Print and shaded views of the part. All mm, measured from the part's lowest x, y and z. A direction names the side the tool comes from. Round coordinates to 2 decimals unless told otherwise and drop trailing zeros. Order: outer loops, then holes, each group sorted by start corner. A loop starts at its lowest first (then second) coordinate and runs counter-clockwise, first axis right, second up. Notation, with made-up numbers: (-32.5, 1.25) - (-16.5, 1.25) arc R31 ccw to (-16.5, 35.25) - close; hole circle Ø3 at (3.5, 82.25). An arc over 180 degrees is marked (long way). Write item = value, one per line.
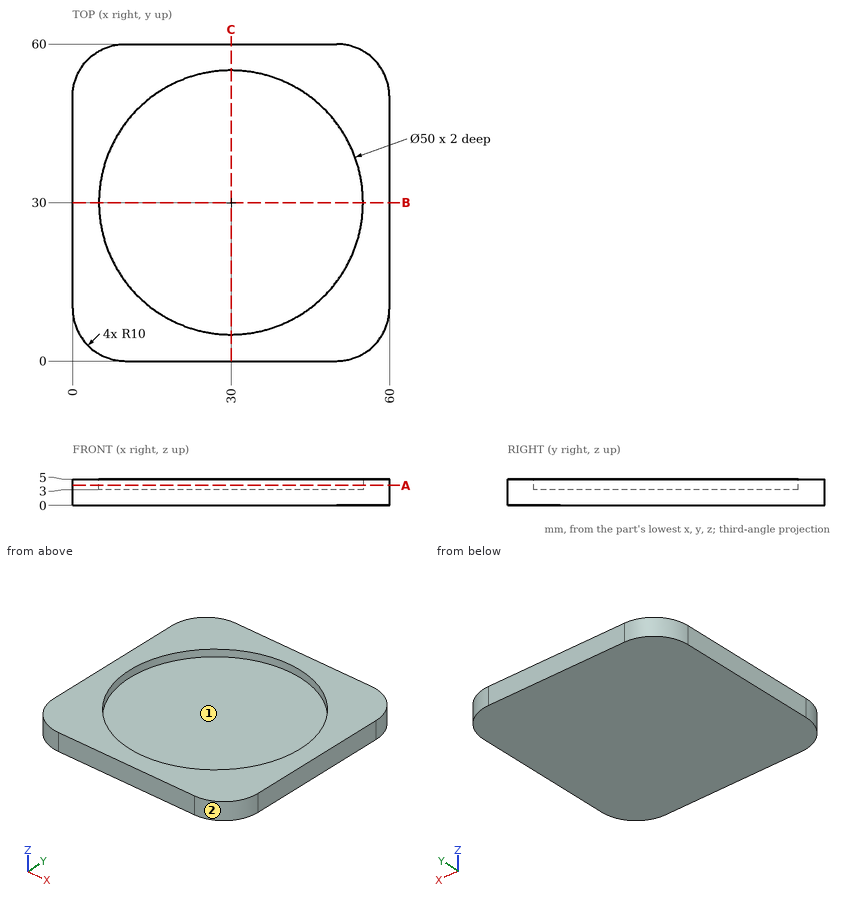
(1) Tool access for the marked faces 1 and 2: list every direction of +Z, -Z, +X, -X, +Y, -Y with a clear straight run to the whole face (end or side of a thin tool).
Solved:
face_1 = +Z
face_2 = +Z, -Z, +X, -Y
(2) Band-saw the part on A-A on z = 3.8. List the corners of the cut face in (x, y), plus the area to 3 significant figures.
Solved:
outline = (0, 10) arc R10 ccw to (10, 0) - (50, 0) arc R10 ccw to (60, 10) - (60, 50) arc R10 ccw to (50, 60) - (10, 60) arc R10 ccw to (0, 50) - close; hole circle Ø50 at (30, 30)
area = 1,550 mm²
(3) Probe line 1 along Y through (x, z) = (30, 3.45); line 2 along Z through (x, y) = (13.5, 42.5); line 3 along X through (y, z) = (20, 4.05). List the from-to ranges inside material, lowest first.
Solved:
line_1 = 0 to 5, 55 to 60
line_2 = 0 to 3
line_3 = 0 to 7.09, 52.91 to 60
(4) Band-saw the part on B-B on y = 30. List the corners of the cut face in (x, z), plus the area to 3 significant figures.
Solved:
outline = (0, 0) - (60, 0) - (60, 5) - (55, 5) - (55, 3) - (5, 3) - (5, 5) - (0, 5) - close
area = 200 mm²
